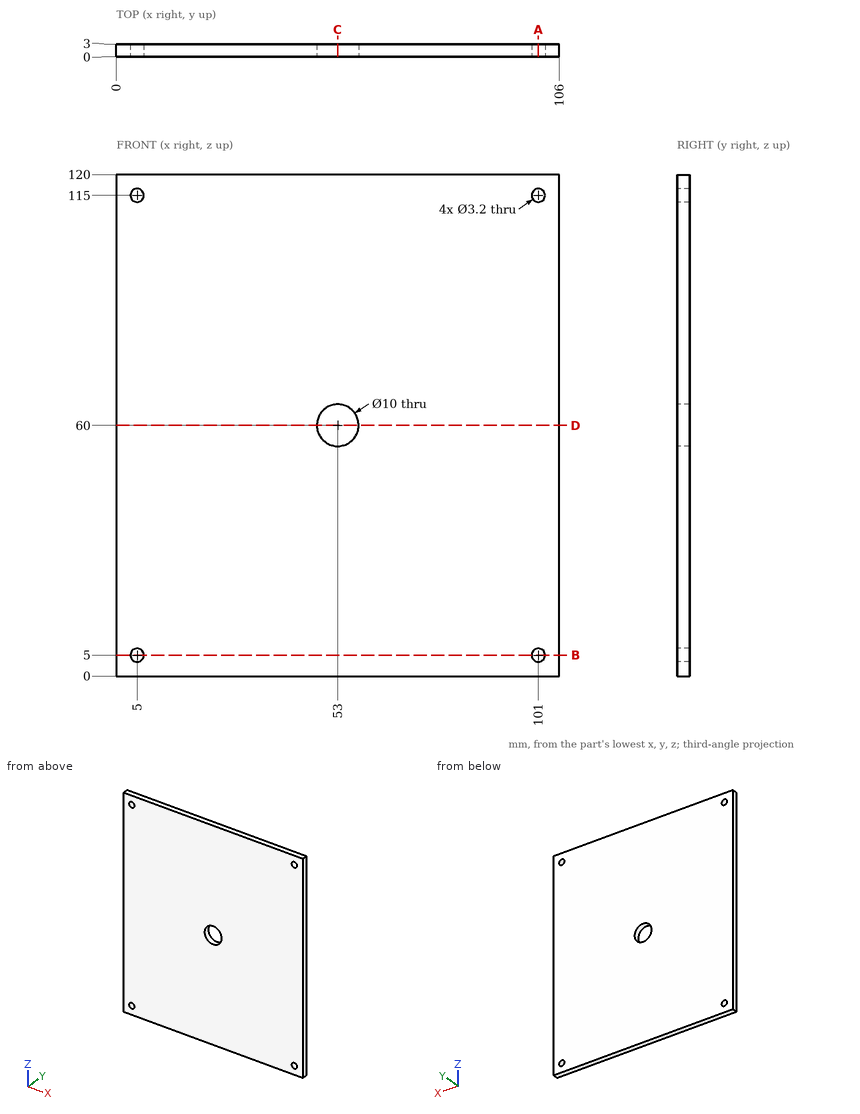
Could you check a few things on this drawing? It's one solid part, dimensions in mm from its lowest x, y, z. Round coordinates to 2 decimals unless told otherwise and drop trailing zeros. Loops run counter-clockwise (first coordinate to the right, second up) from the corner with the lowest first, then second, coordinate; pieces in that order, holes last. Notation, with made-up numbers: (-38, -19) -> (11, -19) arc R15 cw to (11, -8) -> close; hole circle Ø3 at (38, -29.75). An arc over 180 degrees is marked (long way). Answer as CSV lines item,"result".
1. If we section it at B-B on z = 5: Please give me the cut outline in (x, y), plus the area to 3 significant figures.
Final values:
outline,"(0, 0) -> (3.4, 0) -> (3.4, 3) -> (0, 3) -> close; (6.6, 0) -> (99.4, 0) -> (99.4, 3) -> (6.6, 3) -> close; (102.6, 0) -> (106, 0) -> (106, 3) -> (102.6, 3) -> close"
area,"299 mm^2"
2. If we section it at A-A on x = 101: Please give me the cut outline in (y, z).
Final values:
outline,"(0, 0) -> (3, 0) -> (3, 3.4) -> (0, 3.4) -> close; (0, 6.6) -> (3, 6.6) -> (3, 113.4) -> (0, 113.4) -> close; (0, 116.6) -> (3, 116.6) -> (3, 120) -> (0, 120) -> close"
3. If we section it at D-D on z = 60: Please give me the cut outline in (x, y).
Final values:
outline,"(0, 0) -> (48, 0) -> (48, 3) -> (0, 3) -> close; (58, 0) -> (106, 0) -> (106, 3) -> (58, 3) -> close"
4. For pin 1 (3 mm diameter, centred on x = 5, z = 115, fed in from +Y), with a flat end and sliding along its axis, tell me the tip position at first contact or that it passes through.
Final values:
pin 1,"passes through"
5. If we section it at C-C on x = 53: Please give me the cut outline in (y, z).
Final values:
outline,"(0, 0) -> (3, 0) -> (3, 55) -> (0, 55) -> close; (0, 65) -> (3, 65) -> (3, 120) -> (0, 120) -> close"
6. If I drill on L1, parallel to Z at x = 5, y = 1.7; L2, parallel to X at y = 1.35, z = 5; L3, parallel to X at y = 1.75, z = 60, over which ranges is the centre line in solid material (lowest first)?
Final values:
L1,"z = 0 to 3.4, 6.6 to 113.4, 116.6 to 120"
L2,"x = 0 to 3.4, 6.6 to 99.4, 102.6 to 106"
L3,"x = 0 to 48, 58 to 106"
